from build123d import *

# Parameters (mm, degrees)
F0_R     = 6.35
F1_DEPTH = 6.35
F2_R     = 1.524
F3_R     = 1.524


with BuildPart() as f1:
    # F0 (on Top) → F1 (new body, symmetric)
    with BuildSketch(Plane.XY):
        Circle(F0_R)
    extrude(amount=F1_DEPTH, both=True)

    # F2
    f2_edges = [f1.edges().sort_by_distance(p)[0] for p in [
        (-6.35, 0, -6.35),
    ]]
    fillet(f2_edges, radius=F2_R)

    # F3
    f3_edges = [f1.edges().sort_by_distance(p)[0] for p in [
        (-6.35, 0, 6.35),
    ]]
    fillet(f3_edges, radius=F3_R)


solid = f1.part
Source: CAD feature listing. Evaluate the final solid. Frame: model axes, mm. Coordinates: 2 decimals unless noted, no trailing zeros. Loops run counter-clockwise (first coordinate to the right, second up) from the corner with the lowest first, then second, coordinate; pieces in that order, holes last. Notation, with made-up numbers: (87, 20.25) - (139, 20.25) arc R20 cw to (139, 54.25) - close; hole circle Ø4 at (86, 10). An arc over 180 degrees is marked (long way). One line per question, with ' | ' between items.
1) First-contact query: P1, Ø6, axis at x = -5, y = 4, coming from the -Z side; P2, Ø2, axis at x = 2.5, z = -2.5, coming from the +Y side; P3, Ø2, axis at x = 4.5, z = -5, coming from the +Y side; P4, Ø1, axis at y = -3, z = 4, coming from the +X side. Flat tips, straight axial feed; report the tip coordinate or a pass-through.
Report:
P1: stops at z = -6.35 | P2: stops at y = 6.17 | P3: stops at y = 5.29 | P4: stops at x = 5.84
2) Section B-B, the plane z = 5.5. Return loops of the section in (x, y), then the cut area to 3 significant figures.
Report:
outline: circle Ø12.39 at (0, 0) | area: 120 mm²
3) Section A-A, the plane z = -4.5. Return loops of the section in (x, y), then the cut area to 3 significant figures.
Report:
outline: circle Ø12.7 at (0, 0) | area: 127 mm²
4) Line query: line 1 along X through (y, z) = (4.75, 5.5); line 2 along X through (y, z) = (3.5, -5.5); line 3 along Y through (x, z) = (-4.25, 3). Output: solid intervals per line, ascending.
Report:
line 1: x = -3.97 to 3.97 | line 2: x = -5.11 to 5.11 | line 3: y = -4.72 to 4.72
